from build123d import *

# Parameters (mm, degrees)
SKETCH1_W                  = 12.7
SKETCH1_H                  = 63.5
BOSS_EXTRUDE1_DEPTH        = 3.175
F_10_CLEARANCE_HOLE1_D     = 5.6134
F_10_CLEARANCE_HOLE1_DEPTH = 25.4
F_10_CLEARANCE_HOLE1_TIP   = 1.686435499
FILLET1_R                  = 1.5875


with BuildPart() as part:
    # Sketch1 → Boss-Extrude1 (new body)
    with BuildSketch(Plane.XY):
        Rectangle(SKETCH1_W, SKETCH1_H)
    extrude(amount=BOSS_EXTRUDE1_DEPTH)

    # #10 Clearance Hole1
    with Locations(Plane.XY.offset(3.175)):
        with Locations((1.5875, -25.4), (1.5875, 0), (1.5875, 25.4)):
            Hole(F_10_CLEARANCE_HOLE1_D / 2, depth=F_10_CLEARANCE_HOLE1_DEPTH)
            with Locations((0, 0, -(F_10_CLEARANCE_HOLE1_DEPTH + F_10_CLEARANCE_HOLE1_TIP / 2))):  # 118° drill point
                Cone(0, F_10_CLEARANCE_HOLE1_D / 2, F_10_CLEARANCE_HOLE1_TIP, mode=Mode.SUBTRACT)

    # Fillet1
    fillet1_edges = [part.edges().sort_by_distance(p)[0] for p in [
        (6.35, -31.75, 1.5875),
        (-6.35, -31.75, 1.5875),
        (-6.35, 31.75, 1.5875),
        (6.35, 31.75, 1.5875),
    ]]
    fillet(fillet1_edges, radius=FILLET1_R)


solid = part.part
Work out the finished part from the listing and answer in its coordinate system (mm). Give positions to 0.01 mm unless a question says otherwise; leave off trailing zeros. Order: outer loops, then holes, each group sorted by start corner. A loop starts at its lowest first (then second) coordinate and runs counter-clockwise, first axis right, second up. Notation, with made-up numbers: M -3,-18.75 L 15,-18.75 A17 cw 15,2.25 Z; hole C 57.25,57 d1. An arc over 180 degrees is marked long. Return JSON: item names as keys, results as strings.
Q1. Find section B-B, the plane y = 0. Write down the section's boundary in (x, z) (3 decimals).
Answer below:
{"outline": "M -6.35,0 L -1.219,0 L -1.219,3.175 L -6.35,3.175 Z; M 4.394,0 L 6.35,0 L 6.35,3.175 L 4.394,3.175 Z"}
Q2. Find the intervals of material crossed by line 1 along Y through (x, z) = (0, 3.05); line 2 along Y through (x, z) = (4, 0.35); line 3 along X through (y, z) = (-23.5, 2.15), in increasing order. Write a range as [from, to].
Answer below:
{"line 1": "y = [-31.75, -27.71], [-23.09, -2.31], [2.31, 23.09], [27.71, 31.75]", "line 2": "y = [-31.75, -26.83], [-23.97, -1.43], [1.43, 23.97], [26.83, 31.75]", "line 3": "x = [-6.35, -0.48], [3.65, 6.35]"}
Q3. The mould has two halves that part along Y. Classify faces 1 (the face through (-5.9, 31.27, 1.61)), 2 (the face through (0, -31.75, 2)), 3 (the face through (2.2, -28.14, 1.57)): pulls with the +Y half, pulls with the -Y half, needs draft (parallel to the pull), parting line crosses it, or undercut.
Answer below:
{"face 1": "pulls with the +Y half", "face 2": "pulls with the -Y half", "face 3": "undercut"}
Q4. Find section C-C, the plane x = 2. Write down the section's boundary in (y, z) (3 decimals).
Answer below:
{"outline": "M -31.75,0 L -28.176,0 L -28.176,3.175 L -31.75,3.175 Z; M -22.624,0 L -2.776,0 L -2.776,3.175 L -22.624,3.175 Z; M 2.776,0 L 22.624,0 L 22.624,3.175 L 2.776,3.175 Z; M 28.176,0 L 31.75,0 L 31.75,3.175 L 28.176,3.175 Z"}
Q5. Find section A-A, the plane z = 1.35. State how many separate pieces and enclosed holes the cut face has, and give its area (3 significant figures).
Answer below:
{"separate pieces": "1", "enclosed holes": "3", "area": "730 mm^2"}
